Design review of the part built by this model. Coordinates are the model's own, in mm. Face numbers are marked on the shaded views. A direction names the side the tool comes from. Give positions to 0.01 mm unless a question says otherwise; leave off trailing zeros. Write each loop counter-clockwise with the first axis right and the second up, starting at its lowest first coordinate (ties: lowest second). Pieces come first, ordered by that corner, then holes. Notation, with made-up numbers: (9.5, -3) - (56.5, -3) arc R8 cw to (56.5, 4) - close; hole circle Ø1 at (3.5, -0.5). An arc over 180 degrees is marked (long way). Use a Markdown table: item, result. Add a question column.
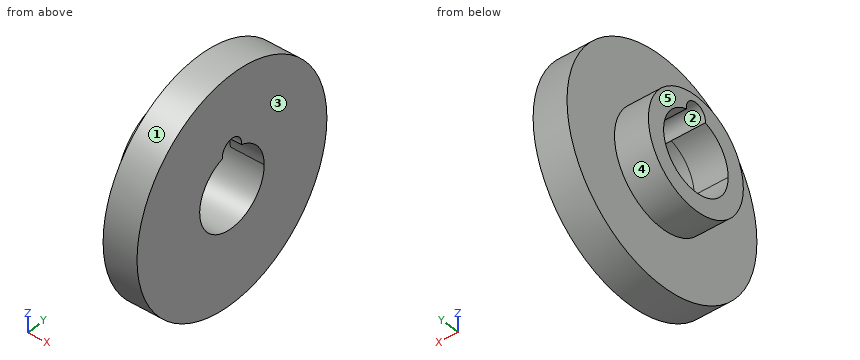
```python
from build123d import *

# Parameters (mm, degrees)
F0_R     = 5
F0_R_2   = 1.7
F1_DEPTH = 1.5
F2_R     = 2.5
F2_R_2   = 1.7
F3_DEPTH = 1.5
F5_D     = 1


with BuildPart() as f1:
    # F0 (on Right) → F1 (new body)
    with BuildSketch(Plane.YZ):
        Circle(F0_R)
        Circle(F0_R_2, mode=Mode.SUBTRACT)
    extrude(amount=F1_DEPTH)

    # F2 (on face) → F3 (join)
    with BuildSketch(Plane(origin=(0, 0, 0), x_dir=(0, -1, 0), z_dir=(-1, 0, 0))):
        Circle(F2_R)
        Circle(F2_R_2, mode=Mode.SUBTRACT)
    extrude(amount=F3_DEPTH)

    # F5 (through all)
    with Locations(Plane(origin=(-1.5, 0, 0), x_dir=(0, -1, 0), z_dir=(-1, 0, 0))):
        with Locations((0, 1.7)):
            Hole(F5_D / 2)


solid = f1.part
```
(1) Insertion check: pin 1 (2.5 mm diameter, centred on y = 0, z = 0, fed in from +X). The pin has a flat end and moves straight along its axis. Give the tip position at first contact, or say it passes through.
(2) Mouldability with a two-part tool opening along Y and no side actions: class the marked faces 1, 2 and 3 as +Y half, -Y half, draft (parallel to the pull), parting line (faces both ways), or undercut.
(3) Add section C-C (x = -0.85). State the section outline as (y, z) points.
(4) Add section A-A (y = 0). State the section outline as (x, z) points.
(5) Add section B-B (z = -0.5). State the section outline as (x, y) points.
(6) Add section D-D (x = 1.15). State the section outline as (y, z) points.
(7) Tool access review of the marked faces 4 and 5: name each direction out of +Z, -Z, +X, -X, +Y, -Y from which nothing blocks a thin tool from reaching the whole face with its end or side.
(8) For line 1 along Z through (x, y) = (-0.4, 0); line 2 along Z through (x, y) = (0.45, 0); line 3 along X through (y, z) = (-3.5, -1.25), list the stretches that pass through material, from the lowest coordinate up.
Answers follow:
| question | item | result |
|---|---|---|
| 1 | pin 1 | through |
| 2 | face 1 | parting line |
| 2 | face 2 | undercut |
| 2 | face 3 | draft |
| 3 | outline | circle Ø5 at (0, 0); hole (-0.49, 1.63) arc R1.7 ccw (long way) to (0.49, 1.63) arc R0.5 ccw (long way) to start |
| 4 | outline | (-1.5, -2.5) - (0, -2.5) - (0, -5) - (1.5, -5) - (1.5, -1.7) - (-1.5, -1.7) - close; (-1.5, 2.2) - (1.5, 2.2) - (1.5, 5) - (0, 5) - (0, 2.5) - (-1.5, 2.5) - close |
| 5 | outline | (-1.5, -2.45) - (0, -2.45) - (0, -4.97) - (1.5, -4.97) - (1.5, -1.62) - (-1.5, -1.62) - close; (-1.5, 1.62) - (1.5, 1.62) - (1.5, 4.97) - (0, 4.97) - (0, 2.45) - (-1.5, 2.45) - close |
| 6 | outline | circle Ø10 at (0, 0); hole (-0.49, 1.63) arc R1.7 ccw (long way) to (0.49, 1.63) arc R0.5 ccw (long way) to start |
| 7 | face 4 | -X |
| 7 | face 5 | +Z, -Z, -X, +Y, -Y |
| 8 | line 1 | -2.5 to -1.7, 2.2 to 2.5 |
| 8 | line 2 | -5 to -1.7, 2.2 to 5 |
| 8 | line 3 | 0 to 1.5 |
